Can you work these out from the model? Positions are in its coordinate system, mm. A direction names the side the tool comes from. Coordinates: 2 decimals unless noted, no trailing zeros. Order: outer loops, then holes, each group sorted by start corner. A loop starts at its lowest first (then second) coordinate and runs counter-clockwise, first axis right, second up. Notation, with made-up numbers: (-20, -38) -> (10, -38) arc R20 ccw to (10, -20) -> close; hole circle Ø1 at (46, 73.5). An arc over 180 degrees is marked (long way). Answer in a Markdown table with one row per item.
```python
from build123d import *

# Parameters (mm, degrees)
F0_W     = 35.7
F0_H     = 24
F0_R     = 2.5
F1_DEPTH = 4
F3_DEPTH = 28
F4_SIZE  = 20
F5_R     = 2.25
F6_DEPTH = 4


with BuildPart() as f1:
    # F0 (on Top) → F1 (new body)
    with BuildSketch(Plane.XY):
        with Locations((17.85, 12)):
            Rectangle(F0_W, F0_H)
        with Locations((9, 12)):
            Circle(F0_R, mode=Mode.SUBTRACT)
        with Locations((26.7, 12)):
            Circle(F0_R, mode=Mode.SUBTRACT)
    extrude(amount=F1_DEPTH)

    # F2 (on face) → F3 (join)
    with BuildSketch(Plane.XY.offset(4)):
        Polygon((31.7, 4), (4, 4), (4, 20), (4, 24), (0, 24), (0, 0), (35.7, 0), (35.7, 24), (31.7, 24), (31.7, 20), align=None)
    extrude(amount=F3_DEPTH)

    # F4
    f4_edges = [f1.edges().sort_by_distance(p)[0] for p in [
        (33.7, 24, 32),
        (2, 24, 32),
    ]]
    chamfer(f4_edges, length=F4_SIZE)

    # F5 (on face) → F6 (cut)
    with BuildSketch(Plane(origin=(0, 4, 0), x_dir=(-1, 0, 0), z_dir=(0, 1, 0))):
        with Locations((-17.85, 23)):
            Circle(F5_R)
        with Locations((-17.85, 13)):
            Circle(F5_R)
    extrude(amount=-F6_DEPTH, mode=Mode.SUBTRACT)


solid = f1.part
```
(1) I need wall thicknesses on line 1 (Z direction, x = 17.85, y = 3.1); line 2 (Y direction, x = 9, z = 1); line 3 (X direction, y = 11.5, z = 2). Which ranges of each line are inside material? Lowest first, please. Write a range as [from, to].
Response values:
| item | result |
|---|---|
| line 1 | [0, 10.75], [15.25, 20.75], [25.25, 32] |
| line 2 | [0, 9.5], [14.5, 24] |
| line 3 | [0, 6.55], [11.45, 24.25], [29.15, 35.7] |
(2) Suppose I cut it at C-C (x = 17.85). Please give me the cut outline in (y, z).
Response values:
| item | result |
|---|---|
| outline | (0, 0) -> (24, 0) -> (24, 4) -> (4, 4) -> (4, 10.75) -> (0, 10.75) -> close; (0, 15.25) -> (4, 15.25) -> (4, 20.75) -> (0, 20.75) -> close; (0, 25.25) -> (4, 25.25) -> (4, 32) -> (0, 32) -> close |
(3) Will these pins go through, and if not, where does the flat tip stop? pin 1 Ø10 at (x, y) = (10, 17.5) entering from +Z; pin 2 Ø5 at (x, z) = (17.85, 23) entering from +Y; pin 3 Ø10 at (y, z) = (15.5, 24) entering from -X; pin 4 Ø3.5 at (x, z) = (17.85, 13) entering from +Y.
Response values:
| item | result |
|---|---|
| pin 1 | z = 4 |
| pin 2 | y = 4 |
| pin 3 | x = 0 |
| pin 4 | through |
(4) Suppose I cut it at B-B (z = 13). Please give me the cut outline in (x, y), and give its area (3 significant figures).
Response values:
| item | result |
|---|---|
| outline | (0, 0) -> (15.6, 0) -> (15.6, 4) -> (4, 4) -> (4, 23) -> (0, 23) -> close; (20.1, 0) -> (35.7, 0) -> (35.7, 23) -> (31.7, 23) -> (31.7, 4) -> (20.1, 4) -> close |
| area | 277 mm2 |
(5) We'd pull the mould along Y, two halves only. Please class faces 1 (the cylindrical face through (8.46, 9.56, 1.97)), 2 (the cylindrical face through (24.7, 10.5, 2)), 3 (the flat face through (2, 14, 22)), 4 (the cylindrical face through (16.812, 2.028, 21.004)): +Y half, -Y half, draft (parallel to the pull), parting line (faces both ways), or undercut.
Response values:
| item | result |
|---|---|
| face 1 | undercut |
| face 2 | undercut |
| face 3 | +Y half |
| face 4 | draft |
(6) Suppose I cut it at A-A (x = 26.7). Please give me the cut outline in (y, z).
Response values:
| item | result |
|---|---|
| outline | (0, 0) -> (9.5, 0) -> (9.5, 4) -> (4, 4) -> (4, 32) -> (0, 32) -> close; (14.5, 0) -> (24, 0) -> (24, 4) -> (14.5, 4) -> close |
(7) On a 3-axis mill with a long thin cutter (end or side, diameter ignored), from which of +Z, -Z, +X, -X, +Y, -Y can I reach the whole of each face in a straight line? I mean faces 5 (the flat face through (18, 24, 3)), 6 (the flat face through (4, 12, 15)). Say none if no direction works.
Response values:
| item | result |
|---|---|
| face 5 | +Z, -Z, +X, -X, +Y |
| face 6 | +Z, +Y |
(8) Suppose I cut it at D-D (y = 6.5). Please give me the cut outline in (x, z).
Response values:
| item | result |
|---|---|
| outline | (0, 0) -> (35.7, 0) -> (35.7, 29.5) -> (31.7, 29.5) -> (31.7, 4) -> (4, 4) -> (4, 29.5) -> (0, 29.5) -> close |
